```python
from build123d import *

# Parameters (mm, degrees)
SKETCH1_W           = 13.5
SKETCH1_H           = 10
BOSS_EXTRUDE1_DEPTH = 10
SKETCH2_R           = 1.6
CUT_EXTRUDE1_DEPTH  = 20.551214796
SKETCH3_R           = 1.6
CUT_EXTRUDE2_DEPTH  = 20.551214796
FILLET1_R           = 3


with BuildPart() as part:
    # Sketch1 → Boss-Extrude1 (new body)
    with BuildSketch(Plane(origin=(0, 0, 0), x_dir=(1, 0, 0), z_dir=(0, 1, 0))):
        with Locations((6.75, -5)):
            Rectangle(SKETCH1_W, SKETCH1_H)
    extrude(amount=BOSS_EXTRUDE1_DEPTH)

    # Sketch2 → Cut-Extrude1 (cut, through all)
    with BuildSketch(Plane.XY.offset(10)):
        with Locations((8.5, 5)):
            Circle(SKETCH2_R)
    extrude(amount=-CUT_EXTRUDE1_DEPTH, mode=Mode.SUBTRACT)

    # Sketch3 → Cut-Extrude2 (cut, through all)
    with BuildSketch(Plane(origin=(0, 10, 0), x_dir=(1, 0, 0), z_dir=(0, 1, 0))):
        with Locations(Location((5, -5, 0), (0, 0, 270))):
            Circle(SKETCH3_R)
    extrude(amount=-CUT_EXTRUDE2_DEPTH, mode=Mode.SUBTRACT)

    # Fillet1
    fillet1_edges = [part.edges().sort_by_distance(p)[0] for p in [
        (13.5, 10, 5),
        (13.5, 0, 5),
        (0, 5, 0),
        (0, 5, 10),
    ]]
    fillet(fillet1_edges, radius=FILLET1_R)


solid = part.part
```
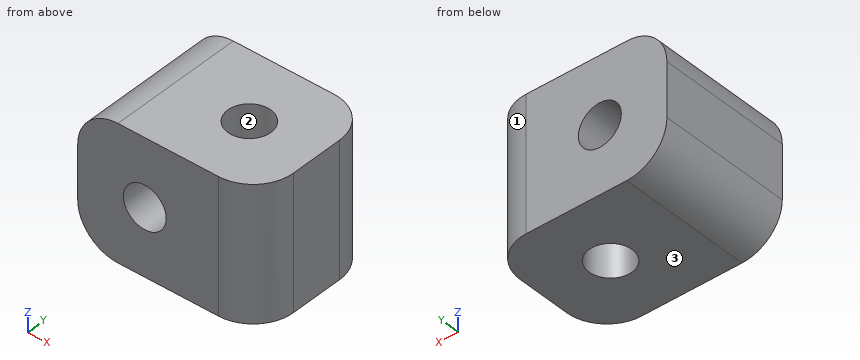
Input: part model. Units: mm. Frame: model coordinates. Face numbers are marked on the shaded views. Give positions to 0.01 mm unless a question says otherwise; leave off trailing zeros. Write each loop counter-clockwise with the first axis right and the second up, starting at its lowest first coordinate (ties: lowest second). Pieces come first, ordered by that corner, then holes. Notation, with made-up numbers: (-0.5, 72) - (37.5, 72) arc R25 ccw to (37.5, 90) - close; hole circle Ø2 at (66, 38). An arc over 180 degrees is marked (long way). Write item = value, one per line. Start each with the question number.
1. Section query B-B, the plane z = 5.75. Output: boundary loops of the cut face in (x, y), then the cut area to 3 significant figures.
2. Mould query, pull axis Y, two halves, no side actions, for the marked faces 1, 2 and 3. Classes: released by +Y, released by -Y, zero draft, split by the parting line, or undercut.
3. Section query A-A, the plane y = 5. Output: boundary loops of the cut face in (x, z), then the cut area to 3 significant figures.
4. First-contact query: pin 1 Ø3 at (y, z) = (7.5, 9) entering from -X; pin 2 Ø3.5 at (x, z) = (5, 5) entering from -Y. Flat tips, straight axial feed; report the tip coordinate or a pass-through.
5. Ray query, L1, parallel to Y at x = 8.5, z = 7.5; L2, parallel to X at y = 5.25, z = 5; L3, parallel to X at y = 4, z = 3.75. Return the intervals inside material, ascending.
6. Section query C-C, the plane x = 8.5. Output: boundary loops of the cut face in (y, z), then the cut area to 3 significant figures.
7. Section query D-D, the plane z = 8.75. Output: boundary loops of the cut face in (x, y).
Check sheet entries:
q1.outline = (0, 0) - (3.59, 0) - (3.59, 10) - (0, 10) - close; (6.41, 0) - (10.5, 0) arc R3 ccw to (13.5, 3) - (13.5, 7) arc R3 ccw to (10.5, 10) - (6.41, 10) - close; hole circle Ø3.2 at (8.5, 5)
q1.area = 94.8 mm2
q2.face_1 = released by +Y
q2.face_2 = undercut
q2.face_3 = zero draft
q3.outline = (0, 3) arc R3 ccw to (3, 0) - (6.9, 0) - (6.9, 10) - (3, 10) arc R3 ccw to (0, 7) - close; (10.1, 0) - (13.5, 0) - (13.5, 10) - (10.1, 10) - close; hole circle Ø3.2 at (5, 5)
q3.area = 91.1 mm2
q4.pin_1 = 0.04
q4.pin_2 = 0
q5.L1 = 0 to 3.4, 6.6 to 10
q5.L2 = 0 to 3.4, 6.6 to 6.92, 10.08 to 13.5
q5.L3 = 0 to 4, 6 to 7.25, 9.75 to 13.5
q6.outline = (0, 0) - (3.4, 0) - (3.4, 10) - (0, 10) - close; (6.6, 0) - (10, 0) - (10, 10) - (6.6, 10) - close
q6.area = 68.0 mm2
q7.outline = (0.56, 0) - (10.5, 0) arc R3 ccw to (13.5, 3) - (13.5, 7) arc R3 ccw to (10.5, 10) - (0.56, 10) - close; hole circle Ø3.2 at (8.5, 5)
